from build123d import *

# Parameters (mm, degrees)
SKETCH_1_R               = 55
EXTRUDE_1_DEPTH          = 3
PATTERN_CIRCULAR_1_COUNT = 6
SKETCH_2_R               = 17.5
CUT_EXTRUDE_1_DEPTH      = 3
CHAMFER_1_SIZE           = 1
CHAMFER_2_SIZE           = 1


with BuildPart() as part:
    # 草图1 → 凸台-拉伸1 (new body)
    with BuildSketch(Plane(origin=(0, 0, 0), x_dir=(1, 0, 0), z_dir=(0, 1, 0))):
        with Locations(Location((0, 0, 0), (0, 0, 270))):
            Circle(SKETCH_1_R)
    extrude(amount=EXTRUDE_1_DEPTH)

    # 草图4 → M8 螺纹孔的螺纹孔钻头1 (revolve, cut)
    with BuildSketch(Plane(origin=(0, 3, -45), x_dir=(0, 0, 1), z_dir=(1, 0, 0))):
        Polygon((0, 0), (0, 18.042926105), (3.4, 16), (3.4, 0), align=None)
    hole_wizard_m8_1 = revolve(axis=Axis((0, 9.35, -45), (0, -1, 0)), mode=Mode.SUBTRACT)

    # 阵列(圆周)1: M8 螺纹孔的螺纹孔钻头1 ×6 about axis
    pattern_circular_1_axis = Axis((0, 0, 0), (0, 1, 0))
    for i in range(1, PATTERN_CIRCULAR_1_COUNT):
        add(hole_wizard_m8_1.rotate(pattern_circular_1_axis, i * 360 / PATTERN_CIRCULAR_1_COUNT), mode=Mode.SUBTRACT)

    # 草图2 → 切除-拉伸1 (cut)
    with BuildSketch(Plane(origin=(0, 3, 0), x_dir=(1, 0, 0), z_dir=(0, 1, 0))):
        with Locations(Location((0, 0, 0), (0, 0, 270))):
            Circle(SKETCH_2_R)
    extrude(amount=-CUT_EXTRUDE_1_DEPTH, mode=Mode.SUBTRACT)

    # 倒角1
    chamfer_1_edges = [part.edges().sort_by_distance(p)[0] for p in [
        (0, 0, -55),
        (0, 3, -55),
    ]]
    chamfer(chamfer_1_edges, length=CHAMFER_1_SIZE)

    # 倒角2
    chamfer_2_edges = [part.edges().sort_by_distance(p)[0] for p in [
        (0, 0, -17.5),
        (0, 3, -17.5),
    ]]
    chamfer(chamfer_2_edges, length=CHAMFER_2_SIZE)


solid = part.part
Geometry: final body of the model. Coordinates: model frame, mm. Round coordinates to 2 decimals unless told otherwise and drop trailing zeros. Loops run counter-clockwise (first coordinate to the right, second up) from the corner with the lowest first, then second, coordinate; pieces in that order, holes last. Notation, with made-up numbers: (43, 24.25) - (102, 24.25) arc R33 cw to (102, 61.25) - close; hole circle Ø1 at (78.5, 78). An arc over 180 degrees is marked (long way). Write each question's results on one line, items separated by ' | '. Start each with the question number.
1) Line query: probe 1 along X at (y, z) = (1.55, 0); probe 2 along X at (y, z) = (2.35, 24); probe 3 along X at (y, z) = (1.35, -22.5). Output: solid intervals per line, ascending. Write a range as [from, to].
2) First-contact query: P1, Ø1.5, axis at y = 1, z = 0.5, coming from the +X side. Flat tip, straight axial feed; report the tip coordinate or a pass-through.
3) Cut plane A-A on z = 0. Return loops of the section in (x, y), then the cut area to 3 significant figures.
4) Cut plane B-B on x = 2. Count the separate pieces of the cut face and the enclosed holes in it, then the cut area to 3 significant figures.
5) Mould query, pull axis X, two halves, no side actions, for faces 1 (the face through (-48.794, 1.493, 25.379)), 2 (the face through (1.021, 1.521, 41.757)), 3 (the face through (-23, 0, -1)). Classes: released by +X, released by -X, zero draft, split by the parting line, or undercut.
Verdict:
1) probe 1: x = [-55, -17.5], [17.5, 55] | probe 2: x = [-49.1, -42.02], [-35.92, 35.92], [42.02, 49.1] | probe 3: x = [-50.19, -42.37], [-35.57, 35.57], [42.37, 50.19]
2) P1: stops at x = 55
3) outline: (-55, 1) - (-54, 0) - (-18.5, 0) - (-17.5, 1) - (-17.5, 2) - (-18.5, 3) - (-54, 3) - (-55, 2) - close; (17.5, 1) - (18.5, 0) - (54, 0) - (55, 1) - (55, 2) - (54, 3) - (18.5, 3) - (17.5, 2) - close | area: 221 mm2
4) separate pieces: 4 | enclosed holes: 0 | area: 188 mm2
5) face 1: split by the parting line | face 2: undercut | face 3: zero draft
